Autodesk Inventor part; units mm, degrees
ref_plane "YZ Plane" through (0, 0, 0) normal (1, 0, 0) x (0, 1, 0)
ref_plane "XZ Plane" through (0, 0, 0) normal (0, 1, 0) x (-1, 0, 0)
ref_plane "XY Plane" through (0, 0, 0) normal (0, 0, 1) x (1, 0, 0)
sketch "Эскиз1" plane through (0, 0, 0) normal (0, 0, 1) x (1, 0, 0)
  line L0 (-10.7121, -2.5) -> (10.5863, -2.5)
  line L1 (10.5863, 2.5) -> (-10.5863, 2.5)
  line L2 (-10.6663, -2.1333) -> (10.6663, 2.1333) construction
  line L3 (10.6663, -2.1333) -> (-10.6663, 2.1333) construction
  arc A0 (6.5383, -2.5) -> (6.5383, 2.5) centre (0, 0) ccw
  line L4 (0, 2.5) -> (0, -2.5) construction
  arc A1 (6.5383, -2.5) -> (6.5383, 2.5) centre (0, 0) ccw
  arc A2 (6.5383, -2.5) -> (6.5383, 2.5) centre (0, 0) ccw
  arc A3 (-6.5383, 2.5) -> (-6.5383, -2.5) centre (0, 0) ccw
  arc A4 (6.5383, -2.5) -> (6.5383, 2.5) centre (0, 0) ccw
  arc A5 (-9.6825, 2.5) -> (-9.6825, -2.5) centre (0, 0) ccw
  arc A6 (9.6825, -2.5) -> (9.6825, 2.5) centre (0, 0) ccw
  arc A7 (-10.5863, 2.5) -> (-10.5863, -2.5) centre (0, 0) ccw
  arc A8 (10.5863, -2.5) -> (10.5863, 2.5) centre (0, 0) ccw
extrude "Выдавливание1" add sketch "Эскиз1" along normal blind 3
extrude "Выдавливание2" add sketch "Эскиз1" against normal blind 8 contours A7 L1 A5 L0 | A5 L1 A3 L0 | A0 L1 A6 L0 | A6 L1 A8 L0
extrude "Выдавливание3" cut sketch "Эскиз1" against normal blind 3 contours A7 L1 A5 L0 | A6 L1 A8 L0
properties part number "move male"
The listing builds one solid part. Answer for the finished solid, in the listing's coordinates (mm). A direction names the side the tool comes from. Round coordinates to 2 decimals unless told otherwise and drop trailing zeros. Loops run counter-clockwise (first coordinate to the right, second up) from the corner with the lowest first, then second, coordinate; pieces in that order, holes last. Notation, with made-up numbers: M 45,13 L 51,13 A19 cw 51,31 Z; hole C 41,22 d4. An arc over 180 degrees is marked long. Write each question's results on one line, items separated by ' | '. Start each with the question number.
1) Find section C-C on x = 1.5. Write down the section's boundary in (y, z), plus the area to 3 significant figures.
2) Straight lines are drawn through the part: probe 1 along Z at (x, y) = (-2.5, 0.1); probe 2 along X at (y, z) = (0.7, -0.75); probe 3 along X at (y, z) = (-2.05, -1.25). For each, find the intervals that lie inside material, in ascending order.
3) Find section A-A on z = -3.25. Write down the section's boundary in (x, y), plus the area to 3 significant figures.
4) Find section D-D on y = -0.85. Write down the section's boundary in (x, z).
5) Which of the six approach directions +Z, -Z, +X, -X, +Y, -Y give full straight-line access (tool end or side, diameter ignored) to faces 4 (the cylindrical face through (-7, 0, -4)), 5 (the cylindrical face through (-10.877, -0.035, -5.535)), 6 (the cylindrical face through (10, 0, -1))?
6) Find section B-B on y = 1.65. Write down the section's boundary in (x, z), plus the area to 3 significant figures.
7) This flat-tipped pin is pushed along its axis until it touches: pin 1 (1.5 mm diameter, centred on y = -0.5, z = -5, fed in from -X). Where does it stop, or does it pass through?
8) Determine the mould class of faces 1 (the cylindrical face through (7, 0, -4)), 2 (the flat face through (0, -2.5, 1)), 3 (the cylindrical face through (-10, 0, -1)) for opening direction X: pulls with the +X half, pulls with the -X half, needs draft (parallel to the pull), parting line crosses it, or undercut.
Final values:
1) outline: M -2.5,0 L 2.5,0 L 2.5,3 L -2.5,3 Z | area: 15.0 mm²
2) probe 1: 0 to 3 | probe 2: -9.98 to -6.96, 6.96 to 9.98 | probe 3: -9.79 to -6.69, 6.69 to 9.79
3) outline: M -10.59,-2.5 L -6.54,-2.5 A7 cw -6.54,2.5 L -10.59,2.5 A10.88 ccw Z; M 6.54,-2.5 L 10.59,-2.5 A10.88 ccw 10.59,2.5 L 6.54,2.5 A7 cw Z | area: 39.3 mm²
4) outline: M -10.84,-8 L -6.95,-8 L -6.95,0 L 6.95,0 L 6.95,-8 L 10.84,-8 L 10.84,-3 L 9.96,-3 L 9.96,0 L 10.84,0 L 10.84,3 L -10.84,3 L -10.84,0 L -9.96,0 L -9.96,-3 L -10.84,-3 Z
5) face 4: -Z | face 5: +Z, -Z, -X | face 6: +X
6) outline: M -10.75,-8 L -6.8,-8 L -6.8,0 L 6.8,0 L 6.8,-8 L 10.75,-8 L 10.75,-3 L 9.86,-3 L 9.86,0 L 10.75,0 L 10.75,3 L -10.75,3 L -10.75,0 L -9.86,0 L -9.86,-3 L -10.75,-3 Z | area: 122 mm²
7) pin 1: x = -10.88
8) face 1: undercut | face 2: needs draft | face 3: pulls with the -X half
